Read the model definition and answer for the solid it produces. Units are mm, in the model's axes. A direction names the side the tool comes from. Give positions to 0.01 mm unless a question says otherwise; leave off trailing zeros. Loops run counter-clockwise (first coordinate to the right, second up) from the corner with the lowest first, then second, coordinate; pieces in that order, holes last. Notation, with made-up numbers: (-33.75, 47.25) - (13.25, 47.25) arc R26 cw to (13.25, 74.25) - close; hole circle Ø6 at (54.25, -36.75). An arc over 180 degrees is marked (long way). Use a Markdown table: item, result. Add a question column.
Item 1: Each of these flat-tipped pins is pushed along its axis until it touches: P1, Ø4, axis at x = 2, y = 15.5, coming from the +Z side; P2, Ø1, axis at y = 39, z = -0.5, coming from the -X side; P3, Ø2, axis at y = 4, z = -2, coming from the -X side. Where does it stop, or does it pass through?
Item 2: Which of the six approach directions +Z, -Z, +X, -X, +Y, -Y give full straight-line access (tool end or side, diameter ignored) to faces 4 (the face through (3, 25, 0)), 5 (the face through (0, 50, 0)), 6 (the face through (0, -2, 0))?
Item 3: Consider probe 1 along Y at (x, z) = (3.5, -1.5); probe 2 along Y at (x, z) = (-2, -0.5); probe 3 along X at (y, z) = (11.5, 0.25). Determine where each line is inside the solid, lowest interval first. Write a range as [from, to].
Item 4: A cutting plane is placed at C-C (y = -0.5). Determine the outline of the cut face in (x, z).
Item 5: A cutting plane is placed at B-B (x = 0). Determine the outline of the cut face in (y, z).
Item 6: For a pull along X with two mould halves and no side action, classify faces 1 (the face through (-1.08, -2.71, -4.88)), 2 (the face through (-0.1, 0, -3.3)), 3 (the face through (2.6, -4, -1.5)) as +X half, -X half, draft (parallel to the pull), parting line (faces both ways), or undercut.
Item 7: A cutting plane is placed at A-A (y = 34). Determine the outline of the cut face in (x, z), plus the area to 3 significant figures.
from build123d import *

# Parameters (mm, degrees)
F0_R     = 5
F1_DEPTH = 6
F3_DEPTH = 4
F6_SIZE  = 0.5
F7_R     = 3
F4_DEPTH = 50
F5_SIZE  = 0.3


with BuildPart() as f1:
    # F0 (on Front) → F1 (new body)
    with BuildSketch(Plane.XZ):
        Circle(F0_R)
    extrude(amount=F1_DEPTH)

    # F2 (on face) → F3 (cut)
    with BuildSketch(Plane.XZ.offset(6)):
        Polygon((3.4639698148, -0.0302179133), (1.7581543879, 2.9847769009), (-1.7058154268, 3.0149948142), (-3.4639698148, 0.0302179133), (-1.7581543879, -2.9847769009), (1.7058154268, -3.0149948142), align=None)
    extrude(amount=-F3_DEPTH, mode=Mode.SUBTRACT)

    # F6
    f6_edges = [f1.edges().sort_by_distance(p)[0] for p in [
        (-5, -6, 0),
        (2.584893, -2, -1.522606),
        (2.611062, -2, 1.477279),
        (0.026169, -2, 2.999886),
        (-2.584893, -2, 1.522606),
        (-2.611062, -2, -1.477279),
        (-0.026169, -2, -2.999886),
        (-2.584893, -6, 1.522606),
        (-2.611062, -6, -1.477279),
        (0.026169, -6, 2.999886),
        (2.584893, -6, -1.522606),
        (2.611062, -6, 1.477279),
        (-0.026169, -6, -2.999886),
    ]]
    chamfer(f6_edges, length=F6_SIZE)

    # F7 (on face) → F4 (join)
    with BuildSketch(Plane(origin=(0, 0, 0), x_dir=(-1, 0, 0), z_dir=(0, 1, 0))):
        Circle(F7_R)
    extrude(amount=F4_DEPTH)

    # F5
    f5_edges = [f1.edges().sort_by_distance(p)[0] for p in [
        (3, 50, 0),
    ]]
    chamfer(f5_edges, length=F5_SIZE)


solid = f1.part
Geometry says:
| question | item | result |
|---|---|---|
| 1 | P1 | z = 3 |
| 1 | P2 | x = -3 |
| 1 | P3 | x = -2.83 |
| 2 | face 4 | +Y |
| 2 | face 5 | +Z, -Z, +X, -X, +Y |
| 2 | face 6 | -Y |
| 3 | probe 1 | [-6, 0] |
| 3 | probe 2 | [-2, 50] |
| 3 | probe 3 | [-2.99, 2.99] |
| 4 | outline | circle Ø10 at (0, 0) |
| 5 | outline | (-6, -4.5) - (-5.5, -5) - (0, -5) - (0, -3) - (49.7, -3) - (50, -2.7) - (50, 2.7) - (49.7, 3) - (0, 3) - (0, 5) - (-5.5, 5) - (-6, 4.5) - (-6, 3.5) - (-5.5, 3) - (-2.5, 3) - (-2, 2.5) - (-2, -2.5) - (-2.5, -3) - (-5.5, -3) - (-6, -3.5) - close |
| 6 | face 1 | parting line |
| 6 | face 2 | draft |
| 6 | face 3 | undercut |
| 7 | outline | circle Ø6 at (0, 0) |
| 7 | area | 28.3 mm² |
